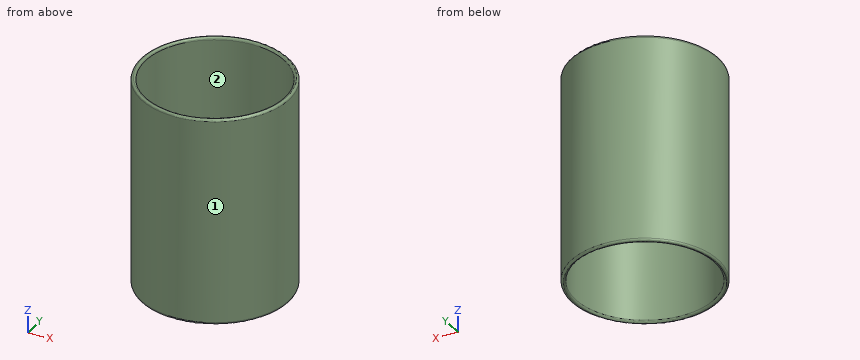
Autodesk Inventor part; units mm, degrees
ref_plane "YZ Plane" through (0, 0, 0) normal (1, 0, 0) x (0, 1, 0)
ref_plane "XZ Plane" through (0, 0, 0) normal (0, 1, 0) x (-1, 0, 0)
ref_plane "XY Plane" through (0, 0, 0) normal (0, 0, 1) x (1, 0, 0)
sketch "Sketch1" plane through (0, 0, 0) normal (0, 0, 1) x (1, 0, 0)
  circle A0 centre (0, 0) radius 42.5
  circle A1 centre (0, 0) radius 40
  dimension "d0" = 85
  dimension "d1" = 80
extrude "Extrusion1" add sketch "Sketch1" along normal blind 120
fillet "Fillet1" radius 1.25 1 edges at (-42.5, 0, 120)
fillet "Fillet2" radius 1.25 1 edges at (-42.5, 0, 0)
fillet "Fillet3" radius 1.25 1 edges at (-40, 0, 0)
fillet "Fillet4" radius 1.25 1 edges at (-40, 0, 120)
equation "\"d0\" = OuterDiameter"
equation "\"d1\" = InnerDiameter"
equation "\"d2\" = height"
equation "\"d4\" = fillet"
equation "\"d5\" = fillet"
equation "\"d6\" = fillet"
equation "\"d7\" = fillet"
equation "\"OuterDiameter\" = InnerDiameter + thickness"
equation "\"InnerDiameter\" = 80"
equation "\"thickness\" = 5"
equation "\"height\" = 120"
equation "\"fillet\" = 0.25 * thickness"
For this review, take the finished solid that the model builds, in its own axes (mm). Face numbers are marked on the shaded views. Coordinates: 2 decimals unless noted, no trailing zeros. Write each loop counter-clockwise with the first axis right and the second up, starting at its lowest first coordinate (ties: lowest second). Pieces come first, ordered by that corner, then holes. Notation, with made-up numbers: (78.5, 32) - (120.5, 32) arc R20 ccw to (120.5, 50) - close; hole circle Ø3 at (61.5, 70). An arc over 180 degrees is marked (long way). Put each result on its own line as item: value.
1. Add section C-C, the plane z = 25.5. Give the boundary of the cut face in (x, y), then the cut area to 3 significant figures.
Values found:
outline: circle Ø85 at (0, 0); hole circle Ø80 at (0, 0)
area: 648 mm²
2. For pin 1 (12 mm diameter, centred on y = 12.5, z = 43, fed in from +X); pin 2 (12 mm diameter, centred on x = 23.5, z = 19, fed in from -Y); pin 3 (1 mm diameter, centred on y = -1, z = 23, fed in from -X), all flat-tipped, find the tip position at first contact; note any pin that passes through.
Values found:
pin 1: x = 42
pin 2: y = -38.73
pin 3: x = -42.5
3. Mouldability with a two-part tool opening along X and no side actions: class the marked faces 1 and 2 as released by +X, released by -X, zero draft, split by the parting line, or undercut.
Values found:
face 1: split by the parting line
face 2: undercut
4. Wall thickness on probe 1 along Y at (x, z) = (0, 45); probe 2 along X at (y, z) = (-1, 41.5); probe 3 along X at (y, z) = (26, 61.5): over which ranges is each line inside the solid? List them lowest first.
Values found:
probe 1: -42.5 to -40, 40 to 42.5
probe 2: -42.49 to -39.99, 39.99 to 42.49
probe 3: -33.62 to -30.4, 30.4 to 33.62
